The model under review builds one solid part; all positions refer to its coordinate system, in mm. A direction names the side the tool comes from. Round coordinates to 2 decimals unless told otherwise and drop trailing zeros. Write each loop counter-clockwise with the first axis right and the second up, starting at its lowest first coordinate (ties: lowest second). Pieces come first, ordered by that corner, then holes. Notation, with made-up numbers: (-25, 18.25) -> (-13, 18.25) arc R35 cw to (-13, 54.25) -> close; hole circle Ø9 at (89.25, 40). An arc over 180 degrees is marked (long way). Return JSON: item names as keys, results as strings. Group by question number.
1. Take a section at C-C, the plane x = 2. Write out the cut boundary in (y, z), then the cut area to 3 significant figures.
2. Mouldability with a two-part tool opening along X and no side actions: class faces 3 (the flat face through (-56, 15, 2)), 4 (the cylindrical face through (60, 28, 2)), 5 (the flat face through (-61, 0, 2)) as pulls with the +X half, pulls with the -X half, needs draft (parallel to the pull), parting line crosses it, or undercut.
3. For line 1 along X through (y, z) = (8, 3); line 2 along Y through (x, z) = (2, 0.5), list the stretches that pass through material, from the lowest coordinate up. Write a range as from..to.
4. Tool access review of faces 1 (the cylindrical face through (-59, 29, 2)), 2 (the flat face through (-1, 0, 2)): name each direction out of +Z, -Z, +X, -X, +Y, -Y from which nothing blocks a thin tool from reaching the whole face with its end or side.
5. Clearance check with flat-ended pins moving along their axes: P1, Ø8, axis at x = -29, y = -7, coming from the -Z side; P2, Ø1.2, axis at x = 27, z = 1.5, coming from the +Y side. State where each tip first meets the part, or that it passes through.
6. Take a section at A-A, the plane y = 6. Write out the cut boundary in (x, z).
from build123d import *

# Parameters (mm, degrees)
F0_W     = 112
F0_H     = 30
F1_DEPTH = 4
F2_R     = 4.99999


# Not quite as in the source:
# - a fillet or chamfer is up to 0.001 mm smaller than in the source, because OpenCascade refuses the exact size


with BuildPart() as f1:
    # F0 (on Top) → F1 (new body)
    with BuildSketch(Plane.XY):
        with Locations((0, -15)):
            Rectangle(F0_W, F0_H)
        Polygon((-56, -30), (-56, 0), (-56, 30), (-61, 30), (-61, -30), align=None)
        Polygon((56, 30), (56, 0), (56, -30), (61, -30), (61, 30), align=None)
    extrude(amount=F1_DEPTH)

    # F2 (radius 5 in the source; OpenCascade refuses exactly that, so slightly less here)
    f2_edges = [f1.edges().sort_by_distance(p)[0] for p in [
        (-61, -30, 2),
        (61, -30, 2),
        (61, 30, 2),
        (-61, 30, 2),
    ]]
    fillet(f2_edges, radius=F2_R)


solid = f1.part
Output:
{
 "1": {"outline": "(-30, 0) -> (0, 0) -> (0, 4) -> (-30, 4) -> close", "area": "120 mm^2"},
 "2": {"face 3": "undercut", "face 4": "pulls with the +X half", "face 5": "pulls with the -X half"},
 "3": {"line 1": "x = -61..-56, 56..61", "line 2": "y = -30..0"},
 "4": {"face 1": "+Z, -Z, -X, +Y", "face 2": "+Z, -Z, +Y"},
 "5": {"P1": "stops at z = 0", "P2": "stops at y = 0"},
 "6": {"outline": "(-61, 0) -> (-56, 0) -> (-56, 4) -> (-61, 4) -> close; (56, 0) -> (61, 0) -> (61, 4) -> (56, 4) -> close"}
}
